The model under review builds one solid part; all positions refer to its coordinate system, in mm. Coordinates: 2 decimals unless noted, no trailing zeros. Write each loop counter-clockwise with the first axis right and the second up, starting at its lowest first coordinate (ties: lowest second). Pieces come first, ordered by that corner, then holes. Notation, with made-up numbers: M 39.25,-9 L 46.25,-9 A24 ccw 46.25,8 Z; hole C -10,64 d11. An arc over 180 degrees is marked long. Answer as a JSON object with one key per item and string values.
```python
from build123d import *

# Parameters (mm, degrees)
F0_W         = 19.05
F0_H         = 19.05
F1_DEPTH     = 19.05
F2_SIZE      = 8.89
F3_T1_DEPTH  = 13.97
F3_T3_DEPTH  = 13.97
F3_T5_DEPTH  = 24.3105122421
F3_T7_DEPTH  = 13.97
F3_S11_W     = 2.54
F3_S11_H     = 2.54
F3_T12_DEPTH = 2.54
F3_S17_W     = 2.54
F3_S17_H     = 2.54
F3_T18_DEPTH = 2.54
F3_S23_W     = 2.54
F3_S23_H     = 2.54
F3_T24_DEPTH = 2.54
F3_S29_W     = 2.54
F3_S29_H     = 2.54
F3_T30_DEPTH = 2.54


# Not quite as in the source:
# - a fillet or chamfer that OpenCascade refuses, or shapes differently, is made with other operations: its cross-section is extruded or revolved along the edge and cut away or added


with BuildPart() as f1:
    # F0 (on Front) → F1 (new body)
    with BuildSketch(Plane.XZ):
        Rectangle(F0_W, F0_H)
    extrude(amount=F1_DEPTH)

    # F2
    f2_edges = [f1.edges().sort_by_distance(p)[0] for p in [
        (0, -19.05, 9.525),
        (0, 0, 9.525),
        (9.525, -9.525, 9.525),
        (-9.525, -9.525, 9.525),
    ]]
    chamfer(f2_edges, length=F2_SIZE)

    # F3: fillet of radius 2.54 on 9 edges, made by hand

    # F3_s2 → F3_t1 (cut)
    with BuildSketch(Plane.XY.offset(-6.985)):
        with BuildLine():
            ThreePointArc((9.525, -16.51), (8.7810512242, -18.3060512242), (6.985, -19.05))
            Line((6.985, -19.05), (9.525, -19.05))
            Line((9.525, -19.05), (9.525, -16.51))
        make_face()
        with BuildLine():
            ThreePointArc((-6.985, 0), (-8.7810512242, -0.7439487758), (-9.525, -2.54))
            Line((-9.525, -2.54), (-9.525, 0))
            Line((-9.525, 0), (-6.985, 0))
        make_face()
        with BuildLine():
            ThreePointArc((-6.985, -19.05), (-8.7810512242, -18.3060512242), (-9.525, -16.51))
            Line((-9.525, -16.51), (-9.525, -19.05))
            Line((-9.525, -19.05), (-6.985, -19.05))
        make_face()
        with BuildLine():
            ThreePointArc((9.525, -2.54), (8.7810512242, -0.7439487758), (6.985, 0))
            Line((6.985, 0), (9.525, 0))
            Line((9.525, 0), (9.525, -2.54))
        make_face()
    extrude(amount=F3_T1_DEPTH, mode=Mode.SUBTRACT)

    # F3_s4 → F3_t3 (cut)
    with BuildSketch(Plane.YZ.offset(-6.985)):
        with BuildLine():
            ThreePointArc((-16.51, -9.525), (-18.3060512242, -8.7810512242), (-19.05, -6.985))
            Line((-19.05, -6.985), (-19.05, -9.525))
            Line((-19.05, -9.525), (-16.51, -9.525))
        make_face()
        with BuildLine():
            ThreePointArc((0, -6.985), (-0.7439487758, -8.7810512242), (-2.54, -9.525))
            Line((-2.54, -9.525), (0, -9.525))
            Line((0, -9.525), (0, -6.985))
        make_face()
    extrude(amount=F3_T3_DEPTH, mode=Mode.SUBTRACT)

    # F3_s6 → F3_t5 (cut)
    with BuildSketch(Plane.XZ.offset(-2.6302561211)):
        with BuildLine():
            ThreePointArc((-9.525, -0.4171024484), (-9.3316540126, 0.5549134698), (-8.7810512242, 1.3789487758))
            Line((-8.7810512242, 1.3789487758), (-9.525, 0.635))
            Line((-9.525, 0.635), (-9.525, -0.4171024484))
        make_face()
    extrude(amount=F3_T5_DEPTH, mode=Mode.SUBTRACT)

    # F3_s8 → F3_t7 (cut)
    with BuildSketch(Plane.XZ.offset(2.54)):
        with BuildLine():
            ThreePointArc((-6.985, -9.525), (-8.7810512242, -8.7810512242), (-9.525, -6.985))
            Line((-9.525, -6.985), (-9.525, -9.525))
            Line((-9.525, -9.525), (-6.985, -9.525))
        make_face()
        with BuildLine():
            ThreePointArc((9.525, -6.985), (8.7810512242, -8.7810512242), (6.985, -9.525))
            Line((6.985, -9.525), (9.525, -9.525))
            Line((9.525, -9.525), (9.525, -6.985))
        make_face()
    extrude(amount=F3_T7_DEPTH, mode=Mode.SUBTRACT)


with BuildPart() as f3_tool10:
    # F3_s11 → F3_t12 (new body)
    with BuildSketch(Plane.YZ.offset(6.985)):
        with Locations((-17.78, -8.255)):
            Rectangle(F3_S11_W, F3_S11_H)
    extrude(amount=F3_T12_DEPTH)

    # F3_s13 → F3_t14 (revolve, cut)
    with BuildSketch(Plane(origin=(6.985, -16.51, -6.985), x_dir=(0, 0.7071067812, 0.7071067812), z_dir=(0, 0.7071067812, -0.7071067812))):
        with BuildLine():
            ThreePointArc((0, -2.54), (2.54, 0), (0, 2.54))
            Line((0, 2.54), (0, -2.54))
        make_face()
    revolve(axis=Axis((6.985, -16.51, -6.985), (1, 0, 0)), mode=Mode.SUBTRACT)


with BuildPart() as f1_1:
    add(f1.part)

    # F3_t9: cut F3_tool10
    add(f3_tool10.part, mode=Mode.SUBTRACT)


with BuildPart() as f3_tool16:
    # F3_s17 → F3_t18 (new body)
    with BuildSketch(Plane.XY.offset(-6.985)):
        with Locations((-8.255, -17.78)):
            Rectangle(F3_S17_W, F3_S17_H)
    extrude(amount=-F3_T18_DEPTH)

    # F3_s19 → F3_t20 (revolve, cut)
    with BuildSketch(Plane(origin=(-6.985, -16.51, -6.985), x_dir=(0.7071067812, 0.7071067812, 0), z_dir=(-0.7071067812, 0.7071067812, 0))):
        with BuildLine():
            ThreePointArc((0, -2.54), (2.54, 0), (0, 2.54))
            Line((0, 2.54), (0, -2.54))
        make_face()
    revolve(axis=Axis((-6.985, -16.51, -6.985), (0, 0, -1)), mode=Mode.SUBTRACT)


with BuildPart() as f1_2:
    add(f1_1.part)

    # F3_t15: cut F3_tool16
    add(f3_tool16.part, mode=Mode.SUBTRACT)


with BuildPart() as f3_tool22:
    # F3_s23 → F3_t24 (new body)
    with BuildSketch(Plane.XZ.offset(2.54)):
        with Locations((-8.255, -8.255)):
            Rectangle(F3_S23_W, F3_S23_H)
    extrude(amount=-F3_T24_DEPTH)

    # F3_s25 → F3_t26 (revolve, cut)
    with BuildSketch(Plane(origin=(-6.985, -2.54, -6.985), x_dir=(0.7071067812, 0, 0.7071067812), z_dir=(-0.7071067812, 0, 0.7071067812))):
        with BuildLine():
            ThreePointArc((0, -2.54), (2.54, 0), (0, 2.54))
            Line((0, 2.54), (0, -2.54))
        make_face()
    revolve(axis=Axis((-6.985, -2.54, -6.985), (0, 1, 0)), mode=Mode.SUBTRACT)


with BuildPart() as f1_3:
    add(f1_2.part)

    # F3_t21: cut F3_tool22
    add(f3_tool22.part, mode=Mode.SUBTRACT)


with BuildPart() as f3_tool28:
    # F3_s29 → F3_t30 (new body)
    with BuildSketch(Plane.YZ.offset(6.985)):
        with Locations((-1.27, -8.255)):
            Rectangle(F3_S29_W, F3_S29_H)
    extrude(amount=F3_T30_DEPTH)

    # F3_s31 → F3_t32 (revolve, cut)
    with BuildSketch(Plane(origin=(6.985, -2.54, -6.985), x_dir=(0, -0.7071067812, 0.7071067812), z_dir=(0, 0.7071067812, 0.7071067812))):
        with BuildLine():
            ThreePointArc((0, -2.54), (2.54, 0), (0, 2.54))
            Line((0, 2.54), (0, -2.54))
        make_face()
    revolve(axis=Axis((6.985, -2.54, -6.985), (1, 0, 0)), mode=Mode.SUBTRACT)


with BuildPart() as f1_4:
    add(f1_3.part)

    # F3_t27: cut F3_tool28
    add(f3_tool28.part, mode=Mode.SUBTRACT)


solid = f1_4.part
```
(1) Add section A-A on z = -2.5. Give the boundary of the cut face in (x, y) (3 decimals).
Results list:
{"outline": "M -9.525,-16.51 A2.54 ccw -6.985,-19.05 L 6.985,-19.05 A2.54 ccw 9.525,-16.51 L 9.525,-2.54 A2.54 ccw 6.985,0 L -6.985,0 A2.54 ccw -9.525,-2.54 Z"}
(2) For pin 1 Ø5 at (x, y) = (-0.5, -15.5) entering from +Z (3 decimals); pin 2 Ø2 at (y, z) = (-10.5, 7) entering from -X; pin 3 Ø2 at (x, y) = (3, -7.5) entering from +Z, all flat-tipped, find the tip position at first contact; note any pin that passes through.
Results list:
{"pin 1": "z = 6.685", "pin 2": "x = -4.16", "pin 3": "z = 8.16"}
(3) Wall thickness on line 1 along Y through (x, z) = (0.75, 6.5) (3 decimals); line 2 along Z through (x, y) = (-5.25, -3.5) (3 decimals); line 3 along Y through (x, z) = (-7, 2.25) (3 decimals): over which ranges is each line inside the solid? List them lowest first. Write a range as from..to.
Results list:
{"line 1": "-13.185..-5.865", "line 2": "-9.525..4.135", "line 3": "-17.435..-1.615"}
(4) Add section B-B on x = 0.25. Give the boundary of the cut face in (y, z) (3 decimals), and give its area (3 significant figures).
Results list:
{"outline": "M -19.05,-6.985 A2.54 ccw -16.51,-9.525 L -2.54,-9.525 A2.54 ccw 0,-6.985 L 0,0.635 L -8.89,9.525 L -10.16,9.525 L -19.05,0.635 Z", "area": "281 mm²"}
(5) Add section D-D on y = -13.25. Give the boundary of the cut face in (x, z) (3 decimals).
Results list:
{"outline": "M -9.525,-6.985 A2.54 ccw -6.985,-9.525 L 6.985,-9.525 A2.54 ccw 9.525,-6.985 L 9.525,0.635 L 3.725,6.435 L -3.725,6.435 L -8.781,1.379 A2.54 ccw -9.525,-0.417 Z"}
(6) Add section C-C on y = -6.5. Give the boundary of the cut face in (x, z) (3 decimals), and give its area (3 significant figures).
Results list:
{"outline": "M -9.525,-6.985 A2.54 ccw -6.985,-9.525 L 6.985,-9.525 A2.54 ccw 9.525,-6.985 L 9.525,0.635 L 3.025,7.135 L -3.025,7.135 L -8.781,1.379 A2.54 ccw -9.525,-0.417 Z", "area": "272 mm²"}
